The listing builds one solid part. Answer for the finished solid, in the listing's coordinates (mm). Face numbers are marked on the shaded views. A direction names the side the tool comes from. Round coordinates to 2 decimals unless told otherwise and drop trailing zeros. Write each loop counter-clockwise with the first axis right and the second up, starting at its lowest first coordinate (ties: lowest second). Pieces come first, ordered by that corner, then holes. Notation, with made-up numbers: (88.5, 77.25) - (144.5, 77.25) arc R17 cw to (144.5, 94.25) - close; hole circle Ø10 at (47, -6.5). An arc over 180 degrees is marked (long way). Use a Markdown table: item, result. Add a question column.
1) Each of these flat-tipped pins is pushed along its axis until it touches: P1, Ø4.5, axis at x = 18, z = 16.5, coming from the +Y side; P2, Ø4.5, axis at x = 17.5, z = 17.78, coming from the +Y side; P3, Ø6, axis at x = 1, z = 11.5, coming from the +Y side; P4, Ø4, axis at y = 48.92, z = -3.1, coming from the -X side. Where does it stop, or does it pass through?
2) A cutting plane is placed at A-A (z = 7.62). Give the vertices of the cut face in (x, y).
3) Find the intervals of material crossed by probe 1 along Y at (x, z) = (13.5, 16.5); probe 2 along Z at (x, y) = (17, 35); probe 3 along X at (y, z) = (18, 9), in increasing order. Write a range as from..to.
4) A cutting plane is placed at D-D (y = 12.5). Give the vertices of the cut face in (x, z), then the cut area to 3 significant figures.
5) Determine the mould class of the marked faces 1, 2 and 3 for opening direction X: +X half, -X half, draft (parallel to the pull), parting line (faces both ways), or undercut.
6) A tool of negligible diameter and unlimited length cuts with its end or side. For the marked faces 4, 5, 6 and 7, from which of +Z, -Z, +X, -X, +Y, -Y can it reach the whole face along a straight path? Write none if from no direction.
7) A cutting plane is placed at C-C (x = 30). Give the vertices of the cut face in (y, z), then the cut area to 3 significant figures.
8) A cutting plane is placed at B-B (y = 6.35). Give the vertices of the cut face in (x, z).
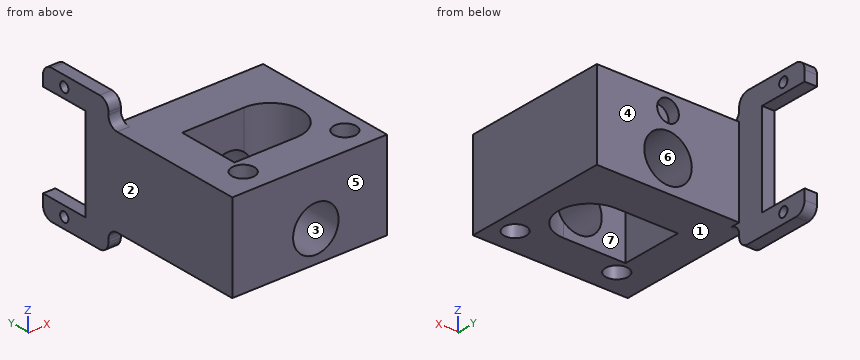
```python
from build123d import *

# Parameters (mm, degrees)
SKETCH2_W            = 35
SKETCH2_H            = 36.068
BOSS_EXTRUDE1_DEPTH  = 21.59
M5_CLEARANCE_HOLE1_D = 5.5
SKETCH13_W           = 22.86
SKETCH13_H           = 15.24
CUT_EXTRUDE3_DEPTH   = 55.699439887
CUT_EXTRUDE1_REACH   = 56.699
SKETCH5_R            = 5.842
BOSS_EXTRUDE2_DEPTH  = 3.048
M2_CLEARANCE_HOLE1_D = 2.4
FILLET2_R            = 2.54
SKETCH11_R           = 2.667
CUT_EXTRUDE2_DEPTH   = 3
SKETCH14_R           = 5.588
CUT_EXTRUDE4_DEPTH   = 64.180572876
FILLET3_R            = 7.62


with BuildPart() as part:
    # Sketch2 → Boss-Extrude1 (new body)
    with BuildSketch(Plane.XY):
        with Locations((17.5, 18.034)):
            Rectangle(SKETCH2_W, SKETCH2_H)
    extrude(amount=BOSS_EXTRUDE1_DEPTH)

    # M5 Clearance Hole1 (through all)
    with Locations(Plane(origin=(0, 0, 0), x_dir=(1, 0, 0), z_dir=(0, 0, -1))):
        with Locations((5, -6.35), (30, -6.35)):
            Hole(M5_CLEARANCE_HOLE1_D / 2)

    # Sketch13 → Cut-Extrude3 (cut, through all)
    with BuildSketch(Plane.XY.offset(21.59)):
        with Locations((17.5, 17.78)):
            Rectangle(SKETCH13_W, SKETCH13_H)
    extrude(amount=-CUT_EXTRUDE3_DEPTH, mode=Mode.SUBTRACT)

    # Sketch5 → Cut-Extrude1 (cut, up to next)
    with BuildSketch(Plane(origin=(0, 36.068, 0), x_dir=(1, 0, 0), z_dir=(0, 1, 0)), mode=Mode.PRIVATE) as cut_extrude1_sk1:
        with Locations(Location((17.5, -7.62, 0), (0, 0, 270))):
            Circle(SKETCH5_R)
    cut_extrude1_tool1 = extrude(cut_extrude1_sk1.sketch, amount=-CUT_EXTRUDE1_REACH, mode=Mode.PRIVATE) & part.part
    add(cut_extrude1_tool1.solids().sort_by_distance((17.5, 36.068, 7.62))[0], mode=Mode.SUBTRACT)

    # Sketch7 → Boss-Extrude2 (add)
    with BuildSketch(Plane.ZY):
        Polygon((-5.715, 55.118), (-5.715, 36.068), (0, 36.068), (0, 0), (21.59, 0), (21.59, 36.068), (27.305, 36.068), (27.305, 55.118), (22.225, 55.118), (22.225, 42.7228), (-0.635, 42.7228), (-0.635, 55.118), align=None)
    extrude(amount=BOSS_EXTRUDE2_DEPTH)

    # M2 Clearance Hole1 (through all)
    with Locations(Plane.ZY.offset(3.048)):
        with Locations((-3.10388, 48.9204), (24.69388, 48.9204)):
            Hole(M2_CLEARANCE_HOLE1_D / 2)

    # Fillet2
    fillet2_edges = [part.edges().sort_by_distance(p)[0] for p in [
        (-1.524, 55.118, -5.715),
        (-1.524, 36.068, -5.715),
        (-1.524, 36.068, 0),
        (-1.524, 36.068, 21.59),
        (-1.524, 36.068, 27.305),
        (-1.524, 55.118, 27.305),
    ]]
    fillet(fillet2_edges, radius=FILLET2_R)

    # Sketch11 → Cut-Extrude2 (cut)
    with BuildSketch(Plane(origin=(0, 36.068, 0), x_dir=(1, 0, 0), z_dir=(0, 1, 0))):
        with Locations(Location((17.5, -17.78, 0), (0, 0, 270))):
            Circle(SKETCH11_R)
    extrude(amount=-CUT_EXTRUDE2_DEPTH, mode=Mode.SUBTRACT)

    # Sketch14 → Cut-Extrude4 (cut, through all)
    with BuildSketch(Plane(origin=(0, 10.16, 0), x_dir=(1, 0, 0), z_dir=(0, 1, 0))):
        with Locations(Location((17.5, -7.62, 0), (0, 0, 270))):
            Circle(SKETCH14_R)
    extrude(amount=-CUT_EXTRUDE4_DEPTH, mode=Mode.SUBTRACT)

    # Fillet3
    # the kernel refuses this fillet: 7.62 mm, written as the material it adds along each edge
    with BuildSketch(Plane(origin=(28.93, 25.4, 21.59), x_dir=(-1, 0, 0), z_dir=(0, 0, -1))) as fillet3_piece_1_section:
        with BuildLine():
            CenterArc((FILLET3_R, -FILLET3_R), FILLET3_R, 90, 90)
            Line((0, -FILLET3_R), (0, 0))
            Line((0, 0), (FILLET3_R, 0))
        make_face()
    fillet3_piece_1 = extrude(amount=21.59, mode=Mode.PRIVATE)
    fillet3_piece_1 = fillet3_piece_1 - Plane(origin=(17.5, 23.659865562, 7.62), x_dir=(0, 0, 1), z_dir=(0, 1, 0)) * Cylinder(5.842, 74, mode=Mode.PRIVATE)
    add(fillet3_piece_1)
    with BuildSketch(Plane(origin=(28.93, 10.16, 21.59), x_dir=(0, 1, 0), z_dir=(0, 0, -1))) as fillet3_piece_2_section:
        with BuildLine():
            CenterArc((FILLET3_R, -FILLET3_R), FILLET3_R, 90, 90)
            Line((0, -FILLET3_R), (0, 0))
            Line((0, 0), (FILLET3_R, 0))
        make_face()
    fillet3_piece_2 = extrude(amount=21.59, mode=Mode.PRIVATE)
    fillet3_piece_2 = fillet3_piece_2 - Plane(origin=(17.5, 11.896400625, 7.62), x_dir=(0, 0, 1), z_dir=(0, 1, 0)) * Cylinder(5.588, 74, mode=Mode.PRIVATE)
    add(fillet3_piece_2)


solid = part.part
```
Entries:
| question | item | result |
|---|---|---|
| 1 | P1 | stops at y = 36.07 |
| 1 | P2 | stops at y = 33.07 |
| 1 | P3 | stops at y = 42.72 |
| 1 | P4 | stops at x = -3.05 |
| 2 | outline | (-3.05, 0) - (11.91, 0) - (11.91, 10.16) - (6.07, 10.16) - (6.07, 25.4) - (11.66, 25.4) - (11.66, 36.07) - (0, 36.07) - (0, 42.72) - (-3.05, 42.72) - close; (23.09, 0) - (35, 0) - (35, 36.07) - (23.34, 36.07) - (23.34, 25.12) arc R7.62 cw to (23.09, 10.37) - close; hole circle Ø5.5 at (5, 6.35); hole circle Ø5.5 at (30, 6.35) |
| 3 | probe 1 | y = 0..10.16, 25.4..36.07 |
| 3 | probe 2 | z = 0..1.8, 13.44..15.16, 20.4..21.59 |
| 3 | probe 3 | x = -3.05..6.07, 28.93..35 |
| 4 | outline | (-3.05, 0) - (6.07, 0) - (6.07, 21.59) - (-3.05, 21.59) - close; (26.8, 0) - (35, 0) - (35, 21.59) - (26.8, 21.59) - close |
| 4 | area | 374 mm² |
| 5 | face 1 | draft |
| 5 | face 2 | -X half |
| 5 | face 3 | undercut |
| 6 | face 4 | +Z, -Z, +X, +Y |
| 6 | face 5 | +Z, -Z, +X, -X, -Y |
| 6 | face 6 | +Y |
| 6 | face 7 | +Z, -Z |
| 7 | outline | (0, 0) - (3.6, 0) - (3.6, 21.59) - (0, 21.59) - close; (9.1, 0) - (36.07, 0) - (36.07, 21.59) - (9.1, 21.59) - close |
| 7 | area | 660 mm² |
| 8 | outline | (-3.05, 0) - (2.25, 0) - (2.25, 21.59) - (-3.05, 21.59) - close; (7.75, 0) - (27.25, 0) - (27.25, 21.59) - (7.75, 21.59) - close; (32.75, 0) - (35, 0) - (35, 21.59) - (32.75, 21.59) - close; hole circle Ø11.18 at (17.5, 7.62) |
